Can you work these out from the model? Positions are in its coordinate system, mm. Round coordinates to 2 decimals unless told otherwise and drop trailing zeros. Order: outer loops, then holes, each group sorted by start corner. A loop starts at its lowest first (then second) coordinate and runs counter-clockwise, first axis right, second up. Notation, with made-up numbers: M -1.75,-24 L 5.25,-24 A16 cw 5.25,0 Z; hole C 40.5,29.25 d10. An arc over 180 degrees is marked long. Answer as a JSON object with one key per item and string values. Group by question number.
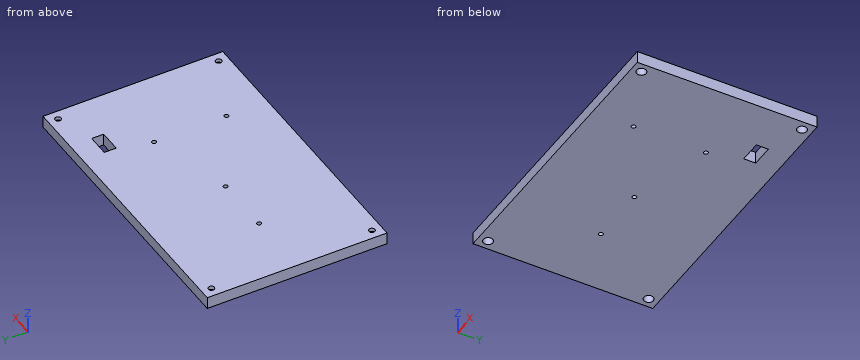
from build123d import *

# Parameters (mm, degrees)
SKETCH_1_W          = 120
SKETCH_1_H          = 75
EXTRUDE_1_DEPTH     = 5
SKETCH_2_R          = 1.25
CUT_EXTRUDE_1_DEPTH = 126.822295322
SKETCH_2_3_R        = 2
CUT_EXTRUDE_2_DEPTH = 3.5
SKETCH_3_W          = 9.2
SKETCH_3_H          = 5
CUT_EXTRUDE_3_DEPTH = 126.822295322
SKETCH_4_R          = 0.9
CUT_EXTRUDE_4_DEPTH = 126.822295322
SKETCH_5_R          = 0.9
CUT_EXTRUDE_5_DEPTH = 126.822295322


with BuildPart() as part:
    # 草图1 → 凸台-拉伸1 (new body)
    with BuildSketch(Plane.XY):
        with Locations((-60, 0)):
            Rectangle(SKETCH_1_W, SKETCH_1_H)
    extrude(amount=EXTRUDE_1_DEPTH)

    # 草图2 → 切除-拉伸1 (cut, through all)
    with BuildSketch(Plane(origin=(0, 0, 0), x_dir=(-1, 0, 0), z_dir=(0, 0, -1))):
        with Locations((4, 33.5)):
            Circle(SKETCH_2_R)
        with Locations((4, -33.5)):
            Circle(SKETCH_2_R)
        with Locations((116, -33.5)):
            Circle(SKETCH_2_R)
        with Locations((116, 33.5)):
            Circle(SKETCH_2_R)
    extrude(amount=-CUT_EXTRUDE_1_DEPTH, mode=Mode.SUBTRACT)

    # 草图2<3> → 切除-拉伸2 (cut)
    with BuildSketch(Plane(origin=(0, 0, 0), x_dir=(-1, 0, 0), z_dir=(0, 0, -1))):
        with Locations((4, 33.5)):
            Circle(SKETCH_2_3_R)
        with Locations((116, 33.5)):
            Circle(SKETCH_2_3_R)
        with Locations((4, -33.5)):
            Circle(SKETCH_2_3_R)
        with Locations((116, -33.5)):
            Circle(SKETCH_2_3_R)
    extrude(amount=-CUT_EXTRUDE_2_DEPTH, mode=Mode.SUBTRACT)

    # 草图3 → 切除-拉伸3 (cut, through all)
    with BuildSketch(Plane(origin=(0, 0, 0), x_dir=(-1, 0, 0), z_dir=(0, 0, -1))):
        with Locations((24.4, 26)):
            Rectangle(SKETCH_3_W, SKETCH_3_H)
    extrude(amount=-CUT_EXTRUDE_3_DEPTH, mode=Mode.SUBTRACT)

    # 草图4 → 切除-拉伸4 (cut, through all)
    with BuildSketch(Plane.XY.offset(5)):
        with Locations((-92.25, 0)):
            Circle(SKETCH_4_R)
        with Locations((-67.75, 0)):
            Circle(SKETCH_4_R)
    extrude(amount=-CUT_EXTRUDE_4_DEPTH, mode=Mode.SUBTRACT)

    # 草图5 → 切除-拉伸5 (cut, through all)
    with BuildSketch(Plane.XY.offset(5)):
        with Locations((-32.75, 9.85)):
            Circle(SKETCH_5_R)
        with Locations((-32.75, -20.35)):
            Circle(SKETCH_5_R)
    extrude(amount=-CUT_EXTRUDE_5_DEPTH, mode=Mode.SUBTRACT)


solid = part.part
Item 1: I need wall thicknesses on line 1 (Y direction, x = -116, z = 1.55); line 2 (Y direction, x = -4, z = 3.85); line 3 (X direction, y = -33, z = 2.2). Which ranges of each line are inside material? Lowest first, please.
Item 2: Suppose I cut it at C-C, the plane y = 33.5. Write out the boundary of the cut face in (x, z), and give its area (4 significant figures).
Item 3: I'm going to push flat-ended pins straight in: pin 1 Ø1.1 at (x, y) = (-92.25, 0) entering from +Z; pin 2 Ø3 at (x, y) = (-4, -33.5) entering from -Z. Where does each tip first touch, or does it pass through?
Item 4: Suppose I cut it at B-B, the plane x = -116. Write out the boundary of the cut face in (y, z), and give its area (4 significant figures).
Item 5: Suppose I cut it at A-A, the plane x = -25.5. Write out the boundary of the cut face in (y, z), and give its area (3 significant figures).
Computed:
{
 "1": {"line 1": "y = -37.5 to -35.5, -31.5 to 31.5, 35.5 to 37.5", "line 2": "y = -37.5 to -34.75, -32.25 to 32.25, 34.75 to 37.5", "line 3": "x = -120 to -117.94, -114.06 to -5.94, -2.06 to 0"},
 "2": {"outline": "M -120,0 L -118,0 L -118,3.5 L -117.25,3.5 L -117.25,5 L -120,5 Z; M -114.75,3.5 L -114,3.5 L -114,0 L -6,0 L -6,3.5 L -5.25,3.5 L -5.25,5 L -114.75,5 Z; M -2.75,3.5 L -2,3.5 L -2,0 L 0,0 L 0,5 L -2.75,5 Z", "area": "564.5 mm^2"},
 "3": {"pin 1": "passes through", "pin 2": "stops at z = 3.5"},
 "4": {"outline": "M -37.5,0 L -35.5,0 L -35.5,3.5 L -34.75,3.5 L -34.75,5 L -37.5,5 Z; M -32.25,3.5 L -31.5,3.5 L -31.5,0 L 31.5,0 L 31.5,3.5 L 32.25,3.5 L 32.25,5 L -32.25,5 Z; M 34.75,3.5 L 35.5,3.5 L 35.5,0 L 37.5,0 L 37.5,5 L 34.75,5 Z", "area": "339.5 mm^2"},
 "5": {"outline": "M -37.5,0 L 23.5,0 L 23.5,5 L -37.5,5 Z; M 28.5,0 L 37.5,0 L 37.5,5 L 28.5,5 Z", "area": "350 mm^2"}
}
